from build123d import *

# Parameters (mm, degrees)
SKETCH1_W                        = 42.5704
SKETCH1_H                        = 75.0824
TOUCHESLEFTSIDE_DEPTH            = 5.08
SKETCH2_W                        = 52.7304
SKETCH2_H                        = 85.2424
SKETCH2_W_2                      = 42.5704
SKETCH2_H_2                      = 75.0824
ENCLOSES_DEPTH                   = 24.13
SKETCH11_W                       = 14.478
SKETCH11_H                       = 29.1084
WIREGAP_DEPTH                    = 5.08
SKETCH6_W                        = 144.78
SKETCH6_H                        = 52.7304
HORIZONTAL_DEPTH                 = 5.08
UPPERDIAGONAL_DEPTH              = 5.08
LOWERDIAGONAL_DEPTH              = 5.08
F_10_START                       = 75.0824
F_10_0_1935_DIAMETER_SLOT1_DEPTH = 5.08
FILLET1_R                        = 2.54
CROSSBEAMSUPPORTHOLES_DEPTH      = 178.945286698
CROSSBEAMSUPPORTHOLES_DEPTH_BACK = 178.945286698
SKETCH12_R                       = 1.778
NUTEMPLACEMENTS1_DEPTH           = 2.54
NUTEMPLACEMENTS2_DEPTH           = 2.54


# Read off the part's stored shape, not the designer's step: #10 (0.1935) Diameter Slot1
with BuildPart() as part:
    # Sketch1 → TouchesLeftSide (new body)
    with BuildSketch(Plane(origin=(0, 0, 0), x_dir=(0, 0, -1), z_dir=(1, 0, 0))):
        with Locations((-21.2852, 37.5412)):
            Rectangle(SKETCH1_W, SKETCH1_H)
    extrude(amount=TOUCHESLEFTSIDE_DEPTH)

    # Sketch2 → Encloses (add)
    with BuildSketch(Plane(origin=(5.08, 0, 0), x_dir=(0, 0, -1), z_dir=(1, 0, 0))):
        with Locations((-21.2852, 37.5412)):
            Rectangle(SKETCH2_W, SKETCH2_H)
        with Locations((-21.2852, 37.5412)):
            Rectangle(SKETCH2_W_2, SKETCH2_H_2, mode=Mode.SUBTRACT)
    extrude(amount=-ENCLOSES_DEPTH)

    # Sketch11 → WireGap (cut)
    with BuildSketch(Plane(origin=(0, 0, 0), x_dir=(1, 0, 0), z_dir=(0, 1, 0))):
        with Locations((-11.811, -19.6342)):
            Rectangle(SKETCH11_W, SKETCH11_H)
    extrude(amount=-WIREGAP_DEPTH, mode=Mode.SUBTRACT)

    # Sketch6 → Horizontal (add)
    with BuildSketch(Plane(origin=(0, 80.1624, 0), x_dir=(1, 0, 0), z_dir=(0, 1, 0))):
        with Locations((77.47, -21.2852)):
            Rectangle(SKETCH6_W, SKETCH6_H)
    extrude(amount=-HORIZONTAL_DEPTH)

    # Sketch7 → UpperDiagonal (add)
    with BuildSketch(Plane.XY.offset(47.6504)):
        Polygon((5.08, -5.08), (5.08, 75.0824), (123.19, 75.0824), align=None)
    extrude(amount=-UPPERDIAGONAL_DEPTH)

    # Sketch8 → LowerDiagonal (add)
    with BuildSketch(Plane(origin=(0, 0, -5.08), x_dir=(-1, 0, 0), z_dir=(0, 0, -1))):
        Polygon((-5.08, -5.08), (-5.08, 75.0824), (-123.19, 75.0824), align=None)
    extrude(amount=-LOWERDIAGONAL_DEPTH)

    # #10 (0.1935) Diameter Slot1 outline → #10 (0.1935) Diameter Slot1 (cut)
    with BuildSketch(Plane(origin=(0, 0, 0), x_dir=(1, 0, 0), z_dir=(0, 1, 0)).offset(F_10_START)):
        with BuildLine():
            Line((127.635, -8.5852), (133.985, -8.5852))
            ThreePointArc((133.985, -8.5852), (137.16, -5.4102), (133.985, -2.2352))
            Line((133.985, -2.2352), (127.635, -2.2352))
            ThreePointArc((127.635, -2.2352), (124.46, -5.4102), (127.635, -8.5852))
        make_face()
        with BuildLine():
            Line((127.635, -40.3352), (133.985, -40.3352))
            ThreePointArc((133.985, -40.3352), (137.16, -37.1602), (133.985, -33.9852))
            Line((133.985, -33.9852), (127.635, -33.9852))
            ThreePointArc((127.635, -33.9852), (124.46, -37.1602), (127.635, -40.3352))
        make_face()
    extrude(amount=F_10_0_1935_DIAMETER_SLOT1_DEPTH, mode=Mode.SUBTRACT)

    # Fillet1
    fillet1_edges = [part.edges().sort_by_distance(p)[0] for p in [
        (123.19, 75.0824, 45.1104),
        (5.08, 35.0012, 42.5704),
        (64.135, 75.0824, 42.5704),
        (5.08, 75.0824, 21.2852),
        (64.135, 75.0824, 0),
        (123.19, 75.0824, -2.54),
        (5.08, 35.0012, 0),
    ]]
    fillet(fillet1_edges, radius=FILLET1_R)

    # Sketch12 → CrossbeamSupportHoles (cut, two sides: drawn at the far end of the back side and taken through both)
    with BuildSketch(Plane.XY.offset(47.6504).offset(-CROSSBEAMSUPPORTHOLES_DEPTH_BACK)):
        with Locations((15.24, 17.164557597)):
            Circle(SKETCH12_R)
        with Locations((15.24, 62.3824)):
            Circle(SKETCH12_R)
    extrude(amount=CROSSBEAMSUPPORTHOLES_DEPTH + CROSSBEAMSUPPORTHOLES_DEPTH_BACK, mode=Mode.SUBTRACT)

    # Sketch13 → NutEmplacements1 (cut)
    with BuildSketch(Plane(origin=(0, 0, 42.5704), x_dir=(-1, 0, 0), z_dir=(0, 0, -1))):
        Polygon((-19.304, 14.818206103), (-15.24, 12.471854609), (-11.176, 14.818206103), (-11.176, 19.510909091), (-15.24, 21.857260585), (-19.304, 19.510909091), align=None)
        Polygon((-15.24, 57.689697012), (-11.176, 60.036048506), (-11.176, 64.728751494), (-15.24, 67.075102988), (-19.304, 64.728751494), (-19.304, 60.036048506), align=None)
    extrude(amount=-NUTEMPLACEMENTS1_DEPTH, mode=Mode.SUBTRACT)

    # Sketch14 → NutEmplacements2 (cut)
    with BuildSketch(Plane.XY):
        Polygon((15.24, 21.857260585), (11.176, 19.510909091), (11.176, 14.818206103), (15.24, 12.471854609), (19.304, 14.818206103), (19.304, 19.510909091), align=None)
        Polygon((15.24, 57.689697012), (19.304, 60.036048506), (19.304, 64.728751494), (15.24, 67.075102988), (11.176, 64.728751494), (11.176, 60.036048506), align=None)
    extrude(amount=-NUTEMPLACEMENTS2_DEPTH, mode=Mode.SUBTRACT)


solid = part.part
Work out the finished part from the listing and answer in its coordinate system (mm). A direction names the side the tool comes from. Give positions to 0.01 mm unless a question says otherwise; leave off trailing zeros. Loops run counter-clockwise (first coordinate to the right, second up) from the corner with the lowest first, then second, coordinate; pieces in that order, holes last. Notation, with made-up numbers: (-14, 60.5) -> (40, 60.5) arc R8 cw to (40, 75.5) -> close; hole circle Ø2 at (45, 68.5). An arc over 180 degrees is marked (long way). Use a Markdown table: item, result. Add a question column.
1. Find the intervals of material crossed by probe 1 along X at (y, z) = (75.5, 5.5); probe 2 along Z at (x, y) = (12.5, 35.5); probe 3 along Y at (x, z) = (15, -3), in increasing order.
2. Section D-D on y = 7.5 is taken. Determine the outline of the cut face in (x, z), and give its area (3 significant figures).
3. Determine the mould class of faces 1 (the flat face through (149.86, 78, 22)), 2 (the flat face through (13, 62, -2.54)), 3 (the flat face through (64.634, 35.34, 45.587)) for opening direction Y: released by +Y, released by -Y, zero draft, split by the parting line, or undercut.
4. Section C-C on x = 48.5 is taken. Determine the outline of the cut face in (y, z).
5. Section B-B on y = 31 is taken. Determine the outline of the cut face in (x, z), and give its area (3 significant figures).
6. Section A-A on z = 14 is taken. Determine the outline of the cut face in (x, y), and give its area (3 significant figures).
7. Flat-ended cylindrical pins translate along their axes: pin 1 Ø5.5 at (x, z) = (-12, 12.5) entering from -Y; pin 2 Ø3 at (y, z) = (63, 44.5) entering from +X; pin 3 Ø5.5 at (x, y) = (15.24, 62.38) entering from +Z; pin 4 Ø2 at (y, z) = (66.5, 36.5) entering from -X. Find the tip coordinate at first contact, or state that the pin passes through.
8. For faces 4 (the flat face through (-4.572, -3, 20)), 5 (the flat face through (-3, 0, 26)), 6 (the flat face through (39, 52, 42.57)), 7 (the flat face through (13, 17, -2.54)), 8 (the cylindrical face through (137.16, 77.59, 5.48)), determine the directions among +Z, -Z, +X, -X, +Y, -Y from which every point of the face is accessible in a straight line to the end or side of a thin tool.
Results below:
| question | item | result |
|---|---|---|
| 1 | probe 1 | x = -19.05 to 124.46, 137.16 to 149.86 |
| 1 | probe 2 | z = -5.08 to 0, 42.57 to 47.65 |
| 1 | probe 3 | y = 1.65 to 15.4, 18.93 to 60.62, 64.14 to 80.16 |
| 2 | outline | (-19.05, -5.08) -> (23.62, -5.08) -> (23.62, 0) -> (7.62, 0) arc R2.54 cw to (5.08, 2.54) -> (5.08, 40.03) arc R2.54 cw to (7.62, 42.57) -> (23.62, 42.57) -> (23.62, 47.65) -> (-19.05, 47.65) -> (-19.05, 42.57) -> (0, 42.57) -> (0, 0) -> (-19.05, 0) -> close |
| 2 | area | 653 mm^2 |
| 3 | face 1 | zero draft |
| 3 | face 2 | undercut |
| 3 | face 3 | released by -Y |
| 4 | outline | (24.39, -5.08) -> (80.16, -5.08) -> (80.16, 47.65) -> (24.39, 47.65) -> (24.39, 42.57) -> (72.54, 42.57) arc R2.54 cw to (75.08, 40.03) -> (75.08, 2.54) arc R2.54 cw to (72.54, 0) -> (24.39, 0) -> close |
| 5 | outline | (-19.05, -5.08) -> (58.24, -5.08) -> (58.24, 0) -> (7.62, 0) arc R2.54 cw to (5.08, 2.54) -> (5.08, 40.03) arc R2.54 cw to (7.62, 42.57) -> (58.24, 42.57) -> (58.24, 47.65) -> (-19.05, 47.65) -> (-19.05, 42.57) -> (0, 42.57) -> (0, 0) -> (-19.05, 0) -> close |
| 5 | area | 1,000 mm^2 |
| 6 | outline | (-19.05, 75.08) -> (0, 75.08) -> (0, 0) -> (-4.57, 0) -> (-4.57, -5.08) -> (5.08, -5.08) -> (5.08, 72.54) arc R2.54 cw to (7.62, 75.08) -> (149.86, 75.08) -> (149.86, 80.16) -> (-19.05, 80.16) -> close |
| 6 | area | 1,290 mm^2 |
| 7 | pin 1 | stops at y = 75.08 |
| 7 | pin 2 | stops at x = 107.6 |
| 7 | pin 3 | stops at z = 47.65 |
| 7 | pin 4 | stops at x = 0 |
| 8 | face 4 | -X, -Y |
| 8 | face 5 | -X |
| 8 | face 6 | +X, -Y |
| 8 | face 7 | none |
| 8 | face 8 | +Y, -Y |
